For this review, take the finished solid that the model builds, in its own axes (mm). Give positions to 0.01 mm unless a question says otherwise; leave off trailing zeros. Order: outer loops, then holes, each group sorted by start corner. A loop starts at its lowest first (then second) coordinate and runs counter-clockwise, first axis right, second up.
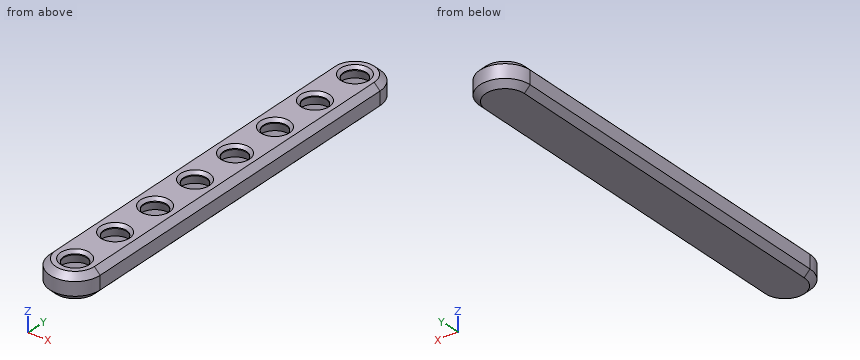
Solid Edge part; units mm, degrees
sketch "Sketch1" plane through (0, 0, 0) normal (0, 0, 1) x (1, 0, 0)
  line L0 (0, 97.5) -> (0, 6.5)
  line L1 (13, 6.5) -> (13, 97.5)
  arc A0 (13, 6.5) -> (0, 6.5) centre (6.5, 6.5) cw
  arc A1 (0, 97.5) -> (13, 97.5) centre (6.5, 97.5) cw
extrude "Protrusion1" add sketch "Sketch1" along normal blind 6.5
sketch "Sketch2" plane through (6.5, 0, 0) normal (1, 0, 0) x (0, 1, 0)
  line L0 (3.5, 5.5) -> (3.5, 6.5)
  line L1 (3.5, 6.5) -> (6.5, 6.5)
  line L2 (6.5, 1) -> (6.5, 6.5)
  line L3 (3.5, 1) -> (6.5, 1)
  line L4 (3.5, 1) -> (2.6811, 3.25)
  line L5 (3.5, 5.5) -> (2.6811, 3.25)
revolve "RevolvedCutout1" cut sketch "Sketch2" angle 360 about axis through (6.5, 6.5, 1) along (0, 0, 1)
chamfer "Chaflán_38" distance 0.75 angle 45 1 edges at (6.5, 3.5, 6.5)
pattern_linear "Pattern1" count 8 spacing 13 along (0, 1, 0) of "RevolvedCutout1", "Chaflán_38"
chamfer "Chaflán_39" distance 1.5 angle 45 8 edges at (13, 52, 6.5) (6.5, 0, 6.5) (0, 52, 6.5) (6.5, 104, 6.5) (13, 52, 0) (6.5, 0, 0) (0, 52, 0) (6.5, 104, 0)
1) Clearance check with flat-ended pins moving along their axes: pin 1 (5 mm diameter, centred on x = 6.5, y = 19.5, fed in from +Z); pin 2 (2 mm diameter, centred on x = 9.5, z = 2.5, fed in from -Y); pin 3 (3 mm diameter, centred on x = 4, z = 2, fed in from -Y). State where each tip first meets the part, or that it passes through.
Answer sheet:
pin 1: stops at z = 1
pin 2: stops at y = 0.32
pin 3: stops at y = 0.08
2) We need section A-A on y = 71.5. Give the boundary of the cut face in (x, z).
Answer sheet:
outline: (0, 1.5) - (1.5, 0) - (11.5, 0) - (13, 1.5) - (13, 5) - (11.5, 6.5) - (10.25, 6.5) - (9.5, 5.75) - (9.5, 5.5) - (10.32, 3.25) - (9.5, 1) - (3.5, 1) - (2.68, 3.25) - (3.5, 5.5) - (3.5, 5.75) - (2.75, 6.5) - (1.5, 6.5) - (0, 5) - close
3) To check wall thickness, follow line 1 (Z direction, x = 9, y = 47); line 2 (X direction, y = 71.5, z = 3.5); line 3 (X direction, y = 44.5, z = 2.25). State the ranges of each line that lie inside material, in increasing order.
Answer sheet:
line 1: z = 0 to 1
line 2: x = 0 to 2.77, 10.23 to 13
line 3: x = 0 to 3.19, 9.81 to 13
